The model under review builds one solid part; all positions refer to its coordinate system, in mm. Face numbers are marked on the shaded views. A direction names the side the tool comes from. Coordinates: 2 decimals unless noted, no trailing zeros. Loops run counter-clockwise (first coordinate to the right, second up) from the corner with the lowest first, then second, coordinate; pieces in that order, holes last. Notation, with made-up numbers: M 39.5,-23 L 52.5,-23 A27 ccw 52.5,4 Z; hole C 62.5,38.5 d2. An arc over 180 degrees is marked long. Use CSV: the item, a comma, the result in double quotes. Start each with the question number.
1. Draft analysis for pull direction Z (two halves, no side actions). For the marked faces 4, 5 and 6, state which applies: +Z half, -Z half, draft (parallel to the pull), parting line (faces both ways), or undercut.
2. Add section C-C, the plane y = 3.6. Write out the cut boundary in (x, z), then the cut area to 3 significant figures.
3. Add section A-A, the plane x = -1. Write out the cut boundary in (y, z), then the cut area to 3 significant figures.
4. Add section D-D, the plane z = -1. Write out the cut boundary in (x, y), then the cut area to 3 significant figures.
5. Clearance check with a flat-ended pin moving along its axis: P1, Ø1.4, axis at y = 4, z = 2, coming from the -X side. State where the tip first meets the part, or that it passes through.
6. Add section B-B, the plane z = -2. Write out the cut boundary in (x, y).
7. Tool access review of the marked faces 1, 2 and 3: name each direction out of +Z, -Z, +X, -X, +Y, -Y from which nothing blocks a thin tool from reaching the whole face with its end or side.
8. For L1, parallel to X at y = 3, z = 0; L2, parallel to X at y = 3.5, z = 0; L3, parallel to Y at x = -3.25, z = 2, list the stretches that pass through material, from the lowest coordinate up.
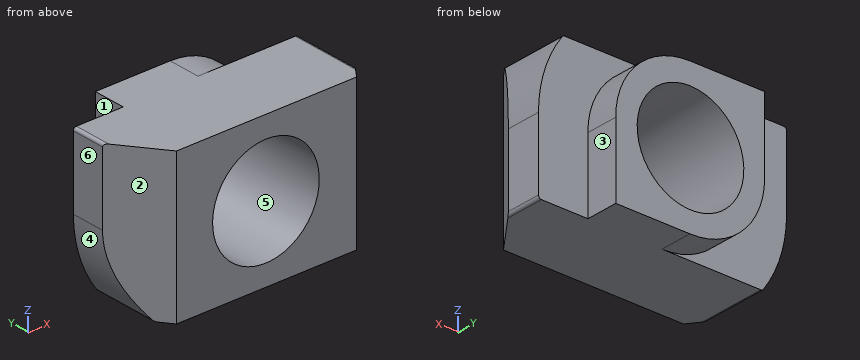
from build123d import *

# Parameters (mm, degrees)
EXTRUDE_1_DEPTH     = 3.2
EXTRUDE_2_DEPTH     = 1.3
CUT_EXTRUDE_1_DEPTH = 4.65
CUT_EXTRUDE_2_REACH = 9.384
SKETCH_4_R          = 2.15


with BuildPart() as part:
    # 草图1 → 凸台-拉伸1 (new body)
    with BuildSketch(Plane(origin=(0, 0, 0), x_dir=(1, 0, 0), z_dir=(0, 1, 0))):
        with BuildLine():
            Line((3.92, -3.012326357), (-4.900543928, -3.012326357))
            ThreePointArc((-4.900543928, -3.012326357), (-4.985396742, -2.97717917), (-5.020543928, -2.892326357))
            Line((-5.020543928, -2.892326357), (-5.020543928, 0))
            ThreePointArc((-5.020543928, 0), (-4.782016181, 1.53758289), (-4.088854807, 2.930631324))
            ThreePointArc((-4.088854807, 2.930631324), (-4.040689897, 2.972567944), (-3.978638656, 2.987673643))
            Line((-3.978638656, 2.987673643), (4.859456072, 2.987673643))
            ThreePointArc((4.859456072, 2.987673643), (4.944308886, 2.952526457), (4.979456072, 2.867673643))
            Line((4.979456072, 2.867673643), (4.979456072, 0))
            ThreePointArc((4.979456072, 0), (4.736196095, -1.552389562), (4.029736524, -2.955957745))
            ThreePointArc((4.029736524, -2.955957745), (3.98168372, -2.997410155), (3.92, -3.012326357))
        make_face()
    extrude(amount=EXTRUDE_1_DEPTH)

    # 草图2 → 凸台-拉伸2 (add)
    with BuildSketch(Plane(origin=(0, 3.2, 0), x_dir=(1, 0, 0), z_dir=(0, 1, 0))):
        with BuildLine():
            Line((0, -3.012326357), (-3.012326357, -3.012326357))
            Line((-3.012326357, -3.012326357), (-3.012326357, 0))
            ThreePointArc((-3.012326357, 0), (-2.128529169, 2.12133825), (0, 2.987673643))
            Line((0, 2.987673643), (2.987673643, 2.987673643))
            Line((2.987673643, 2.987673643), (2.987673643, 0))
            ThreePointArc((2.987673643, 0), (2.12133825, -2.128529169), (0, -3.012326357))
        make_face()
    extrude(amount=EXTRUDE_2_DEPTH)

    # 草图3 → 切除-拉伸1 (cut, symmetric)
    with BuildSketch(Plane.XY):
        Polygon((5.020543928, 0), (3.63, 0), (5.020543928, 1.845314119), align=None)
        Polygon((-3.63, 0), (-5.020543928, 1.845314119), (-5.020543928, 0), align=None)
    extrude(amount=CUT_EXTRUDE_1_DEPTH, both=True, mode=Mode.SUBTRACT)

    # 草图4 → 切除-拉伸2 (cut, up to next)
    with BuildSketch(Plane(origin=(0, 4.5, 0), x_dir=(1, 0, 0), z_dir=(0, 1, 0)), mode=Mode.PRIVATE) as cut_extrude_2_sk1:
        with Locations(Location((-0.024551835, 0, 0), (0, 0, 270))):
            Circle(SKETCH_4_R)
    cut_extrude_2_tool1 = extrude(cut_extrude_2_sk1.sketch, amount=-CUT_EXTRUDE_2_REACH, mode=Mode.PRIVATE) & part.part
    add(cut_extrude_2_tool1.solids().sort_by_distance((-0.024552, 4.5, 0))[0], mode=Mode.SUBTRACT)


solid = part.part
Computed:
1,face 4,"-Z half"
1,face 5,"undercut"
1,face 6,"draft"
2,outline,"M -3.01,0 A2.99 ccw 0,-2.99 L 2.99,-2.99 L 2.99,0 A2.99 ccw 0,3.01 L -3.01,3.01 Z; hole C -0.02,0 d4.3"
2,area,"17.6 mm^2"
3,outline,"M 0,-2.99 L 3.2,-2.99 L 3.2,-2.82 L 4.5,-2.82 L 4.5,-1.92 L 0,-1.92 Z; M 0,1.92 L 4.5,1.92 L 4.5,3.01 L 0,3.01 Z"
3,area,"9.54 mm^2"
4,outline,"M -4.92,1.71 L -3.63,0 L -1.93,0 L -1.93,4.5 L -2.84,4.5 L -2.84,3.2 L -4.92,3.2 Z; M 1.88,0 L 3.63,0 L 4.98,1.79 L 4.98,3.2 L 2.99,3.2 L 2.99,4.5 L 1.88,4.5 Z"
4,area,"19.8 mm^2"
5,P1,"stops at x = -3.01"
6,outline,"M -4.61,1.3 L -3.63,0 L -0.81,0 L -0.81,4.5 L -2.24,4.5 L -2.24,3.2 L -4.61,3.2 Z; M 0.76,0 L 3.63,0 L 4.98,1.79 L 4.98,3.2 L 2.99,3.2 L 2.99,4.5 L 0.76,4.5 Z"
7,face 1,"+Z, -Z, -X, +Y"
7,face 2,"+Z, -Z, -X, -Y"
7,face 3,"+Z, -Z, +X, +Y"
8,L1,"x = -5.02 to -2.17, 2.13 to 4.98"
8,L2,"x = -3.01 to -2.17, 2.13 to 2.99"
8,L3,"y = 0 to 3.2"
